Design review of the part built by this model. Coordinates are the model's own, in mm. A direction names the side the tool comes from. Coordinates: 2 decimals unless noted, no trailing zeros. Write each loop counter-clockwise with the first axis right and the second up, starting at its lowest first coordinate (ties: lowest second). Pieces come first, ordered by that corner, then holes. Notation, with made-up numbers: (23, 43.5) - (42, 43.5) arc R35 cw to (42, 82.5) - close; hole circle Ø2 at (-7.5, 43.5). An arc over 180 degrees is marked (long way). Answer as a JSON object with one key per item and string values.
```python
from build123d import *

# Parameters (mm, degrees)
SKETCH3_W           = 38.1
SKETCH3_H           = 101.6
SKETCH3_W_2         = 31.75
SKETCH3_H_2         = 95.25
BOSS_EXTRUDE1_DEPTH = 114.3
CUT_EXTRUDE1_DEPTH  = 158.602855304
CUT_EXTRUDE2_REACH  = 159.603
SKETCH6_R           = 2.4003
SKETCH6_R_2         = 3.175
CUT_EXTRUDE3_REACH  = 159.603
SKETCH7_R           = 2.5146
SKETCH7_R_2         = 6.35


with BuildPart() as part:
    # Sketch3 → Boss-Extrude1 (new body)
    with BuildSketch(Plane.XY):
        with Locations((19.05, 50.8)):
            Rectangle(SKETCH3_W, SKETCH3_H)
        with Locations((19.05, 50.8)):
            Rectangle(SKETCH3_W_2, SKETCH3_H_2, mode=Mode.SUBTRACT)
    extrude(amount=BOSS_EXTRUDE1_DEPTH)

    # Sketch5 → Cut-Extrude1 (cut, through all)
    with BuildSketch(Plane.ZY):
        Polygon((0, 101.6), (0, 6.35), (25.4, 101.6), align=None)
        Polygon((66.675, 88.9), (38.1, 28.575), (38.1, 0), (114.3, 0), (114.3, 88.9), align=None)
    extrude(amount=-CUT_EXTRUDE1_DEPTH, mode=Mode.SUBTRACT)

    # Sketch6 → Cut-Extrude2 (cut, up to next)
    with BuildSketch(Plane.XZ, mode=Mode.PRIVATE) as cut_extrude2_sk1:
        with Locations(Location((31.75, 6.35, 0), (0, 0, 270))):
            Circle(SKETCH6_R)
    cut_extrude2_tool1 = extrude(cut_extrude2_sk1.sketch, amount=-CUT_EXTRUDE2_REACH, mode=Mode.PRIVATE) & part.part
    # Sketch6 → Cut-Extrude2 (cut, up to next)
    with BuildSketch(Plane.XZ, mode=Mode.PRIVATE) as cut_extrude2_sk2:
        with Locations(Location((6.35, 6.35, 0), (0, 0, 270))):
            Circle(SKETCH6_R)
    cut_extrude2_tool2 = extrude(cut_extrude2_sk2.sketch, amount=-CUT_EXTRUDE2_REACH, mode=Mode.PRIVATE) & part.part
    # Sketch6 → Cut-Extrude2 (cut, up to next)
    with BuildSketch(Plane.XZ, mode=Mode.PRIVATE) as cut_extrude2_sk3:
        with Locations(Location((19.05, 19.05, 0), (0, 0, 270))):
            Circle(SKETCH6_R_2)
    cut_extrude2_tool3 = extrude(cut_extrude2_sk3.sketch, amount=-CUT_EXTRUDE2_REACH, mode=Mode.PRIVATE) & part.part
    add(cut_extrude2_tool1.solids().sort_by_distance((31.75, 0, 6.35))[0], mode=Mode.SUBTRACT)
    add(cut_extrude2_tool2.solids().sort_by_distance((6.35, 0, 6.35))[0], mode=Mode.SUBTRACT)
    add(cut_extrude2_tool3.solids().sort_by_distance((19.05, 0, 19.05))[0], mode=Mode.SUBTRACT)

    # Sketch7 → Cut-Extrude3 (cut, up to next)
    with BuildSketch(Plane(origin=(0, 101.6, 0), x_dir=(1, 0, 0), z_dir=(0, 1, 0)), mode=Mode.PRIVATE) as cut_extrude3_sk1:
        with Locations(Location((6.35, -101.6, 0), (0, 0, 270))):
            Circle(SKETCH7_R)
    cut_extrude3_tool1 = extrude(cut_extrude3_sk1.sketch, amount=-CUT_EXTRUDE3_REACH, mode=Mode.PRIVATE) & part.part
    # Sketch7 → Cut-Extrude3 (cut, up to next)
    with BuildSketch(Plane(origin=(0, 101.6, 0), x_dir=(1, 0, 0), z_dir=(0, 1, 0)), mode=Mode.PRIVATE) as cut_extrude3_sk2:
        with Locations(Location((31.75, -101.6, 0), (0, 0, 270))):
            Circle(SKETCH7_R)
    cut_extrude3_tool2 = extrude(cut_extrude3_sk2.sketch, amount=-CUT_EXTRUDE3_REACH, mode=Mode.PRIVATE) & part.part
    # Sketch7 → Cut-Extrude3 (cut, up to next)
    with BuildSketch(Plane(origin=(0, 101.6, 0), x_dir=(1, 0, 0), z_dir=(0, 1, 0)), mode=Mode.PRIVATE) as cut_extrude3_sk3:
        with Locations(Location((19.05, -101.6, 0), (0, 0, 270))):
            Circle(SKETCH7_R_2)
    cut_extrude3_tool3 = extrude(cut_extrude3_sk3.sketch, amount=-CUT_EXTRUDE3_REACH, mode=Mode.PRIVATE) & part.part
    # Sketch7 → Cut-Extrude3 (cut, up to next)
    with BuildSketch(Plane(origin=(0, 101.6, 0), x_dir=(1, 0, 0), z_dir=(0, 1, 0)), mode=Mode.PRIVATE) as cut_extrude3_sk4:
        with BuildLine():
            Line((25.4, -41.275), (25.4, -76.2))
            ThreePointArc((25.4, -76.2), (19.05, -82.55), (12.7, -76.2))
            Line((12.7, -76.2), (12.7, -41.275))
            ThreePointArc((12.7, -41.275), (19.05, -34.925), (25.4, -41.275))
        make_face()
    cut_extrude3_tool4 = extrude(cut_extrude3_sk4.sketch, amount=-CUT_EXTRUDE3_REACH, mode=Mode.PRIVATE) & part.part
    add(cut_extrude3_tool1.solids().sort_by_distance((6.35, 101.6, 101.6))[0], mode=Mode.SUBTRACT)
    add(cut_extrude3_tool2.solids().sort_by_distance((31.75, 101.6, 101.6))[0], mode=Mode.SUBTRACT)
    add(cut_extrude3_tool3.solids().sort_by_distance((19.05, 101.6, 101.6))[0], mode=Mode.SUBTRACT)
    add(cut_extrude3_tool4.solids().sort_by_distance((19.05, 101.6, 58.7375))[0], mode=Mode.SUBTRACT)


solid = part.part
```
(1) To check wall thickness, follow line 1 (X direction, y = 0.75, z = 6.35); line 2 (X direction, y = 100.85, z = 101.6); line 3 (Y direction, x = 27, z = 33) (3 decimals). State the ranges of each line that lie inside material, in increasing order. Write a range as from..to.
Solved:
{"line 1": "x = 0..3.95, 8.75..29.35, 34.15..38.1", "line 2": "x = 0..3.84, 8.86..12.7, 25.4..29.24, 34.26..38.1", "line 3": "y = 0..3.175, 98.425..101.6"}
(2) Take a section at A-A, the plane x = 19.05. Write out the cut boundary in (y, z) (3 decimals), and give its area (3 significant figures).
Solved:
{"outline": "(0, 0) - (3.175, 0) - (3.175, 15.875) - (0, 15.875) - close; (0, 22.225) - (3.175, 22.225) - (3.175, 38.1) - (0, 38.1) - close; (98.425, 24.553) - (101.6, 25.4) - (101.6, 34.925) - (98.425, 34.925) - close; (98.425, 82.55) - (101.6, 82.55) - (101.6, 95.25) - (98.425, 95.25) - close; (98.425, 107.95) - (101.6, 107.95) - (101.6, 114.3) - (98.425, 114.3) - close", "area": "193 mm^2"}
(3) For pin 1 (6 mm diameter, centred on x = 31.75, z = 101.6, fed in from -Y) (3 decimals); pin 2 (5.5 mm diameter, centred on x = 6.35, z = 6.35, fed in from -Y); pin 3 (1.6 mm diameter, centred on x = 36, z = 88, fed in from -Y); pin 4 (8.5 mm diameter, centred on x = 19.05, z = 19.05, fed in from +Y) (3 decimals), all flat-tipped, find the tip position at first contact; note any pin that passes through.
Solved:
{"pin 1": "stops at y = 98.425", "pin 2": "stops at y = 0", "pin 3": "stops at y = 88.9", "pin 4": "stops at y = 3.175"}
(4) Take a section at B-B, the plane z = 101.6. Write out the cut boundary in (x, y) (3 decimals).
Solved:
{"outline": "(0, 88.9) - (3.175, 88.9) - (3.175, 98.425) - (3.835, 98.425) - (3.835, 101.6) - (0, 101.6) - close; (8.865, 98.425) - (12.7, 98.425) - (12.7, 101.6) - (8.865, 101.6) - close; (25.4, 98.425) - (29.235, 98.425) - (29.235, 101.6) - (25.4, 101.6) - close; (34.265, 98.425) - (34.925, 98.425) - (34.925, 88.9) - (38.1, 88.9) - (38.1, 101.6) - (34.265, 101.6) - close"}
(5) Take a section at C-C, the plane x = 6.35. Write out the cut boundary in (y, z) (3 decimals).
Solved:
{"outline": "(0, 0) - (3.175, 0) - (3.175, 3.95) - (0, 3.95) - close; (0, 8.75) - (3.175, 8.75) - (3.175, 38.1) - (0, 38.1) - close; (98.425, 24.553) - (101.6, 25.4) - (101.6, 99.085) - (98.425, 99.085) - close; (98.425, 104.115) - (101.6, 104.115) - (101.6, 114.3) - (98.425, 114.3) - close"}
(6) Take a section at D-D, the plane y = 67. Write out the cut boundary in (x, z) (3 decimals).
Solved:
{"outline": "(0, 16.173) - (3.175, 16.173) - (3.175, 56.301) - (0, 56.301) - close; (34.925, 16.173) - (38.1, 16.173) - (38.1, 56.301) - (34.925, 56.301) - close"}
(7) Tool access review of faces 4 (the face through (3.175, 61, 44)), 5 (the face through (19.19, 100.03, 82.55)), 6 (the face through (19, 100, 114.3)), 7 (the face through (18.91, 100.035, 34.927)), 8 (the face through (36, 88.9, 91)): name each direction out of +Z, -Z, +X, -X, +Y, -Y from which nothing blocks a thin tool from reaching the whole face with its end or side.
Solved:
{"face 4": "+Z, -Z", "face 5": "+Y, -Y", "face 6": "+Z, +X, -X, +Y, -Y", "face 7": "+Y", "face 8": "+Z, +X, -X, -Y"}
(8) The part is to be moulded in two halves that separate along Z. For faces 1 (the face through (1.565, 59.16, 52.588)), 2 (the face through (8.73, 1.57, 6.66)), 3 (the face through (34.925, 61, 44)), say which applies: pulls with the +Z half, pulls with the -Z half, needs draft (parallel to the pull), parting line crosses it, or undercut.
Solved:
{"face 1": "pulls with the +Z half", "face 2": "undercut", "face 3": "needs draft"}
